CAD build for the part. Positions are in the model's coordinates, mm. Round coordinates to 2 decimals unless told otherwise and drop trailing zeros. Loops run counter-clockwise (first coordinate to the right, second up) from the corner with the lowest first, then second, coordinate; pieces in that order, holes last.
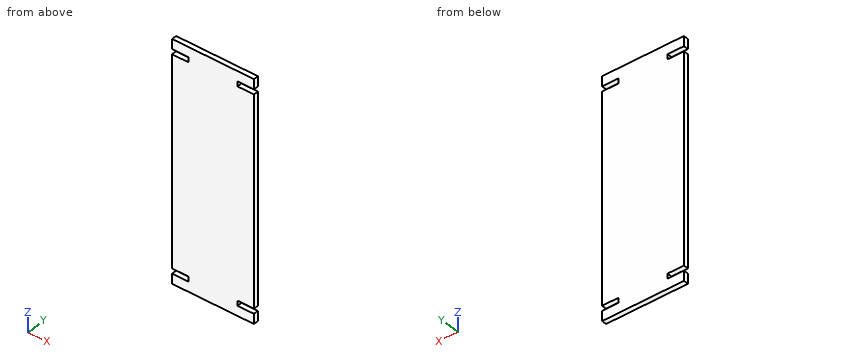
from build123d import *

# Parameters (mm, degrees)
SKETCH1_W            = 100
SKETCH1_H            = 288
BOSS_EXTRUDE1_DEPTH  = 6
SKETCH2_W            = 20
SKETCH2_H            = 6
CUT_EXTRUDE1_DEPTH   = 305.926220585
LPATTERN1_COUNT      = 2
LPATTERN1_PITCH      = 258
LPATTERN1_COUNT_DIR2 = 2
LPATTERN1_PITCH_DIR2 = 80


with BuildPart() as part:
    # Sketch1 → Boss-Extrude1 (new body)
    with BuildSketch(Plane(origin=(0, 0, 0), x_dir=(1, 0, 0), z_dir=(0, 1, 0))):
        with Locations((-50, 144)):
            Rectangle(SKETCH1_W, SKETCH1_H)
    extrude(amount=BOSS_EXTRUDE1_DEPTH)

    # Sketch2 → Cut-Extrude1 (cut, through all)
    with BuildSketch(Plane(origin=(0, 6, 0), x_dir=(1, 0, 0), z_dir=(0, 1, 0))):
        with Locations((-90, 273)):
            Rectangle(SKETCH2_W, SKETCH2_H)
    cut_extrude1 = extrude(amount=-CUT_EXTRUDE1_DEPTH, mode=Mode.SUBTRACT)

    # LPattern1: Cut-Extrude1 2 × 2
    with Locations(*[(j * LPATTERN1_PITCH_DIR2, 0, i * LPATTERN1_PITCH) for i in range(LPATTERN1_COUNT) for j in range(LPATTERN1_COUNT_DIR2) if (i, j) != (0, 0)]):
        add(cut_extrude1, mode=Mode.SUBTRACT)


solid = part.part
Item 1: Flat gauge pins, fed straight in: P1, Ø3, axis at y = 2, z = -14, coming from the +X side; P2, Ø1.8, axis at y = 2.5, z = -15.5, coming from the -X side. Where does each tip first touch, or does it go through?
Verdict:
P1: stops at x = -20
P2: stops at x = -80
Item 2: Wall check: L1, parallel to Z at x = -12.5, y = 0.95; L2, parallel to X at y = 3.15, z = -271. Give the ranges that are in metal, low to high.
Verdict:
L1: z = -288 to -276, -270 to -18, -12 to 0
L2: x = -80 to -20
Item 3: Cut at A-A (x = -7). List the corners of the cut face in (y, z).
Verdict:
outline: (0, -288) - (6, -288) - (6, -276) - (0, -276) - close; (0, -270) - (6, -270) - (6, -18) - (0, -18) - close; (0, -12) - (6, -12) - (6, 0) - (0, 0) - close
Item 4: Cut at B-B (y = 3.8). List the corners of the cut face in (x, z), plus the area to 3 significant figures.
Verdict:
outline: (-100, -288) - (0, -288) - (0, -276) - (-20, -276) - (-20, -270) - (0, -270) - (0, -18) - (-20, -18) - (-20, -12) - (0, -12) - (0, 0) - (-100, 0) - (-100, -12) - (-80, -12) - (-80, -18) - (-100, -18) - (-100, -270) - (-80, -270) - (-80, -276) - (-100, -276) - close
area: 28,300 mm2
